For this review, use the dimensioned drawing (mm, ordinates from the lowest corner) and the shaded views. A direction names the side the tool comes from. Round coordinates to 2 decimals unless told otherwise and drop trailing zeros. Write each loop counter-clockwise with the first axis right and the second up, starting at its lowest first coordinate (ties: lowest second). Pieces come first, ordered by that corner, then holes. Notation, with made-up numbers: M 60.25,8 L 97.25,8 A25 ccw 97.25,27 Z; hole C 86,11 d10. An arc over 180 degrees is marked long. Use one line per item in the form item = value. Start each with the question number.
Item 1: Draft analysis for pull direction Z (two halves, no side actions). For the marked faces 1, 2 and 3, state which applies: released by +Z, released by -Z, zero draft, split by the parting line, or undercut.
Item 2: For line 1 (Y direction, x = 16, z = 76); line 2 (Z direction, x = 7, y = 7); line 3 (X direction, y = 9, z = 47.5), list the stretches that pass through material, from the lowest coordinate up. Write a range as [from, to].
Item 3: Add section B-B (y = 40). State the section outline as (x, z) points.
Item 4: Add section D-D (y = 60). State the section outline as (x, z) points.
Item 5: Add section A-A (x = 10). State the section outline as (y, z) points.
Item 6: For the marked faces 4 and 5, list the 3-axis set-ups (+Z, -Z, +X, -X, +Y, -Y) from which the entire face can be reached by the end or side of a thin tool; tool diameter is ignored.
Item 7: For P1, Ø20.5, axis at y = 22, z = 28, coming from the -X side; P2, Ø12, axis at x = 28, z = 21, coming from the +Y side; P3, Ø14.5, axis at x = 8.5, y = 40, coming from the -Z side; P4, Ø2, axis at x = 36, y = 46, coming from the +Z side, all flat-tipped, find the tip position at first contact; note any pin that passes through.
Item 8: Add section C-C (x = 16). State the section outline as (y, z) points, and give its area (3 significant figures).
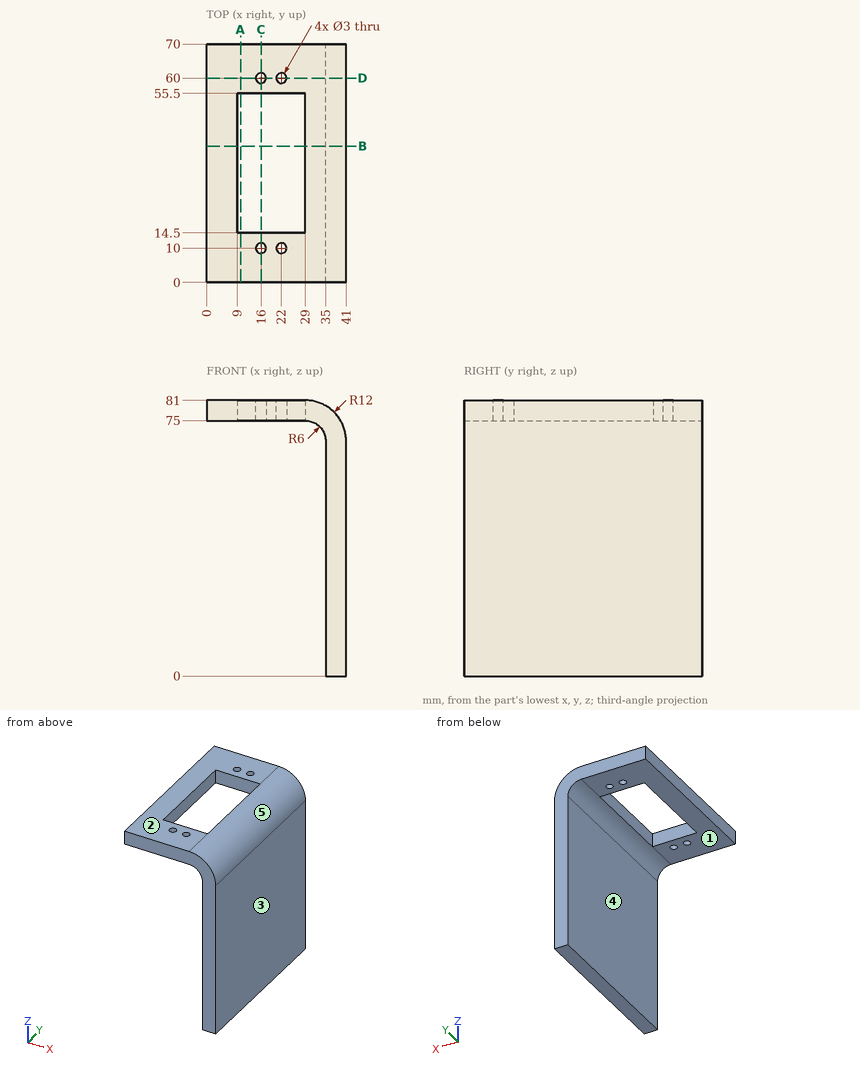
Calculated:
q1.face_1 = released by -Z
q1.face_2 = released by +Z
q1.face_3 = zero draft
q2.line_1 = [0, 8.5], [11.5, 14.5], [55.5, 58.5], [61.5, 70]
q2.line_2 = [75, 81]
q2.line_3 = [35, 41]
q3.outline = M 0,75 L 9,75 L 9,81 L 0,81 Z; M 29,75 A6 cw 35,69 L 35,0 L 41,0 L 41,69 A12 ccw 29,81 Z
q4.outline = M 0,75 L 14.5,75 L 14.5,81 L 0,81 Z; M 17.5,75 L 20.5,75 L 20.5,81 L 17.5,81 Z; M 23.5,75 L 29,75 A6 cw 35,69 L 35,0 L 41,0 L 41,69 A12 ccw 29,81 L 23.5,81 Z
q5.outline = M 0,75 L 14.5,75 L 14.5,81 L 0,81 Z; M 55.5,75 L 70,75 L 70,81 L 55.5,81 Z
q6.face_4 = -Z, -X, +Y, -Y
q6.face_5 = +Z, +X, +Y, -Y
q7.P1 = 35
q7.P2 = through
q7.P3 = 75
q7.P4 = 79.39
q8.outline = M 0,75 L 8.5,75 L 8.5,81 L 0,81 Z; M 11.5,75 L 14.5,75 L 14.5,81 L 11.5,81 Z; M 55.5,75 L 58.5,75 L 58.5,81 L 55.5,81 Z; M 61.5,75 L 70,75 L 70,81 L 61.5,81 Z
q8.area = 138 mm^2
